Read the model definition and answer for the solid it produces. Units are mm, in the model's axes. A direction names the side the tool comes from. Coordinates: 2 decimals unless noted, no trailing zeros. Write each loop counter-clockwise with the first axis right and the second up, starting at its lowest first coordinate (ties: lowest second). Pieces come first, ordered by that corner, then holes. Notation, with made-up numbers: (-34.5, -14) -> (-8.5, -14) arc R21 ccw to (-8.5, 11) -> close; hole circle Ø7 at (67.25, 89.5). An arc over 180 degrees is marked (long way). One line per item, written item: value. Start each with the question number.
1. Find section C-C, the plane z = 4.5. State how many separate pieces and enclosed holes the cut face has, and give its area (3 significant figures).
2. Find section D-D, the plane x = 21. Write down the section's boundary in (y, z), and give its area (3 significant figures).
3. For a pull along X with two mould halves and no side action, classify faces 3 (the flat face through (86.5, 26.6, 15.2)), 4 (the flat face through (-30, 3, 17)), 5 (the flat face through (-86.5, 26.6, 15.2)) as pulls with the +X half, pulls with the -X half, needs draft (parallel to the pull), parting line crosses it, or undercut.
4. Given P1, Ø10, axis at y = 27, z = 6, coming from the +X side; P2, Ø1.6, axis at y = 3.5, z = 8.5, coming from the -X side; P3, Ø1, axis at x = 135.5, z = 9, coming from the +Y side; P4, Ø1, axis at x = 93.5, z = 4.5, coming from the -Y side, each flat-ended and moving along its own axis, determine where each tip first touches the part or whether it passes through.
5. Find section A-A, the plane y = 37. Write down the section's boundary in (x, z), and give its area (3 significant figures).
6. For faces 1 (the flat face through (-102, 48, 16)), 2 (the flat face through (-6, 4, 15.2)), determine the directions among +Z, -Z, +X, -X, +Y, -Y from which every point of the face is accessible in a straight line to the end or side of a thin tool.
7. Find section B-B, the plane x = 103. Write down the section's boundary in (y, z).
8. Consider line 1 along X through (y, z) = (4.5, 14.5); line 2 along Y through (x, z) = (93, 2.75); line 3 along Z through (x, y) = (-90.5, 11.5). Determine where each line is inside the solid, lowest interval first.
```python
from build123d import *

# Parameters (mm, degrees)
F0_W     = 44
F0_H     = 44
F1_DEPTH = 17
F2_W     = 2
F2_H     = 2
F2_W_2   = 4
F2_H_2   = 4
F2_W_3   = 3.5
F3_DEPTH = 20
F4_W     = 4
F4_H     = 38
F4_W_2   = 86.5
F4_H_2   = 2
F5_DEPTH = 2
F7_R     = 3
F8_R     = 3
F9_DEPTH = 15


with BuildPart() as f1:
    # F0 (on Top) → F1 (new body)
    with BuildSketch(Plane.XY):
        Polygon((-138.5, 0), (-90.5, 0), (0, 0), (0, 2), (-90.5, 2), (-90.5, 48), (-138.5, 48), align=None)
        with Locations((-114.5, 24)):
            Rectangle(F0_W, F0_H, mode=Mode.SUBTRACT)
    extrude(amount=F1_DEPTH)

    # F2 (on face) → F3 (join)
    with BuildSketch(Plane.XY.offset(17)):
        with Locations((-135.5, 3)):
            Rectangle(F2_W, F2_H)
        with Locations((-135.5, 45)):
            Rectangle(F2_W, F2_H)
        with Locations((-93.5, 3)):
            Rectangle(F2_W, F2_H)
        with Locations((-93.5, 45)):
            Rectangle(F2_W, F2_H)
        with Locations((-88.5, 46)):
            Rectangle(F2_W_2, F2_H_2)
        with Locations((-88.5, 4)):
            Rectangle(F2_W_2, F2_H_2)
        with Locations((-30.25, 3)):
            Rectangle(F2_W_3, F2_H)
    extrude(amount=-F3_DEPTH)

    # F4 (on face) → F5 (join)
    with BuildSketch(Plane.XY.offset(17)):
        with Locations((-88.5, 25)):
            Rectangle(F4_W, F4_H)
        with Locations((-43.25, 3)):
            Rectangle(F4_W_2, F4_H_2)
    extrude(amount=-F5_DEPTH)

    # F6: F1 across face


with BuildPart() as f1_1:
    add(f1.part)
    add(f1.part.mirror(Plane(origin=(0, 1.2105263158, 9.2894736842), x_dir=(0, 1, 0), z_dir=(1, 0, 0))))

    # F7
    f7_edges = [f1_1.edges().sort_by_distance(p)[0] for p in [
        (-138.5, 0, 8.5),
        (138.5, 0, 8.5),
    ]]
    fillet(f7_edges, radius=F7_R)

    # F8
    f8_edges = [f1_1.edges().sort_by_distance(p)[0] for p in [
        (-138.5, 48, 8.5),
        (138.5, 48, 8.5),
    ]]
    fillet(f8_edges, radius=F8_R)

    # F9 (cut): a face of the model
    f9_faces = [f1_1.faces().sort_by_distance(p)[0] for p in [
        (-138.2188719153, 24, 0),
    ]]
    extrude(f9_faces, amount=-F9_DEPTH, mode=Mode.SUBTRACT)


solid = f1_1.part
```
Answer block:
1. separate pieces: 14
1. enclosed holes: 0
1. area: 110 mm2
2. outline: (0, 15) -> (4, 15) -> (4, 17) -> (0, 17) -> close
2. area: 8.00 mm2
3. face 3: undercut
3. face 4: needs draft
3. face 5: undercut
4. P1: passes through
4. P2: stops at x = -136.5
4. P3: stops at y = 46
4. P4: stops at y = 2
5. outline: (-138.5, 15) -> (-136.5, 15) -> (-136.5, 17) -> (-138.5, 17) -> close; (-92.5, 15) -> (-86.5, 15) -> (-86.5, 17) -> (-92.5, 17) -> close; (86.5, 15) -> (92.5, 15) -> (92.5, 17) -> (86.5, 17) -> close; (136.5, 15) -> (138.5, 15) -> (138.5, 17) -> (136.5, 17) -> close
5. area: 32.0 mm2
6. face 1: +Z, -Z, +X, -X, +Y
6. face 2: +Z, -Z, +Y
7. outline: (0, 15) -> (2, 15) -> (2, 17) -> (0, 17) -> close; (46, 15) -> (48, 15) -> (48, 17) -> (46, 17) -> close
8. line 1: x = -90.5 to -86.5, 86.5 to 90.5
8. line 2: y = 2 to 4, 44 to 46
8. line 3: z = 15 to 17
